Solid Edge part; units mm, degrees
sketch "Sketch1" plane through (0, 0, 0) normal (0, 0, 1) x (1, 0, 0)
  circle A0 centre (0, 0) radius 30
extrude "Ajout_matière_1" add sketch "Sketch1" along normal blind 30
sketch "Sketch2" plane through (0, 0, 30) normal (0, 0, 1) x (1, 0, 0)
  circle A0 centre (0, 0) radius 13.25
extrude "Enlèvement_matière_1" cut sketch "Sketch2" against normal blind 8
sketch "Sketch3" plane through (0, 0, 0) normal (0, 0, 1) x (1, 0, 0)
  circle A0 centre (0, 0) radius 3.6
extrude "Ajout_matière_2" add sketch "Sketch3" along normal blind 35
sketch "Sketch4" plane through (0, 0, 35) normal (0, 0, 1) x (1, 0, 0)
  line L0 (-2.01, 1.445) -> (2.01, 1.445)
  arc A0 (2.01, 1.445) -> (2.01, -1.445) centre (-0.2708, 0) cw
  line L1 (2.01, -1.445) -> (-2.01, -1.445)
  arc A1 (-2.01, -1.445) -> (-2.01, 1.445) centre (0.2708, 0) cw
  dimension "D1" = 2.01
extrude "Enlèvement_matière_2" cut sketch "Sketch4" against normal blind 28.188
properties material "Acier S235"
Could you check a few things on this model? Use its own coordinates, in mm. A direction names the side the tool comes from. Coordinates: 2 decimals unless noted, no trailing zeros. Write each loop counter-clockwise with the first axis right and the second up, starting at its lowest first coordinate (ties: lowest second). Pieces come first, ordered by that corner, then holes. Notation, with made-up numbers: (56, -16.5) - (68, -16.5) arc R33 cw to (68, 15.5) - close; hole circle Ø7 at (-19, -3.75). An arc over 180 degrees is marked (long way). Write item = value, one per line.
1) Please list where these lines run through material, in increasing order: line 1 (Y direction, x = 0, z = 27.5) (3 decimals); line 2 (X direction, y = 2, z = 24.5); line 3 (Z direction, x = 0.5, y = 22). Write a range as [from, to].
Result set:
line_1 = [-30, -13.25], [-3.6, -1.445], [1.445, 3.6], [13.25, 30]
line_2 = [-29.93, -13.1], [-2.99, 2.99], [13.1, 29.93]
line_3 = [0, 30]
2) Will these pins go through, and if not, where does the flat tip stop? pin 1 Ø10 at (x, y) = (14, 6.5) entering from +Z; pin 2 Ø6 at (y, z) = (-15.5, 14.5) entering from +X; pin 3 Ø3 at (x, z) = (-0.5, 15.5) entering from -Y.
Result set:
pin_1 = 30
pin_2 = 27.27
pin_3 = -30
3) Suppose I cut it at B-B on y = 0. Please give me the cut outline in (x, z).
Result set:
outline = (-30, 0) - (30, 0) - (30, 30) - (13.25, 30) - (13.25, 22) - (3.6, 22) - (3.6, 35) - (2.43, 35) - (2.43, 6.81) - (-2.43, 6.81) - (-2.43, 35) - (-3.6, 35) - (-3.6, 22) - (-13.25, 22) - (-13.25, 30) - (-30, 30) - close
4) We'd pull the mould along X, two halves only. Please class faces 1 (the cylindrical face through (-29.97, -1.32, 14.79)), 2 (the cylindrical face through (7.123, 11.172, 26.056)), 3 (the flat face through (0, 0, 0)): +X half, -X half, draft (parallel to the pull), parting line (faces both ways), or undercut.
Result set:
face_1 = parting line
face_2 = undercut
face_3 = draft
5) Suppose I cut it at C-C on x = 0. Please give me the cut outline in (y, z) (3 decimals), plus the area to 3 significant figures.
Result set:
outline = (-30, 0) - (30, 0) - (30, 30) - (13.25, 30) - (13.25, 22) - (3.6, 22) - (3.6, 35) - (1.445, 35) - (1.445, 6.812) - (-1.445, 6.812) - (-1.445, 35) - (-3.6, 35) - (-3.6, 22) - (-13.25, 22) - (-13.25, 30) - (-30, 30) - close
area = 1,600 mm2
6) For faces 4 (the flat face through (0, -2, 35)), 5 (the flat face through (3, -3, 22)), which set-ups out of +Z, -Z, +X, -X, +Y, -Y let a thin tool reach every point of the face, with its end or its side?
Result set:
face_4 = +Z, +X, -X, +Y, -Y
face_5 = +Z
7) Suppose I cut it at D-D on y = -7.5. Please give me the cut outline in (x, z), plus the area to 3 significant figures.
Result set:
outline = (-29.05, 0) - (29.05, 0) - (29.05, 30) - (10.92, 30) - (10.92, 22) - (-10.92, 22) - (-10.92, 30) - (-29.05, 30) - close
area = 1,570 mm2
8) Suppose I cut it at A-A on z = 24. Please give me the cut outline in (x, y) (3 decimals).
Result set:
outline = circle Ø60 at (0, 0); circle Ø7.2 at (0, 0); hole circle Ø26.5 at (0, 0); hole (-2.01, -1.445) - (2.01, -1.445) arc R2.7 ccw to (2.01, 1.445) - (-2.01, 1.445) arc R2.7 ccw to start
